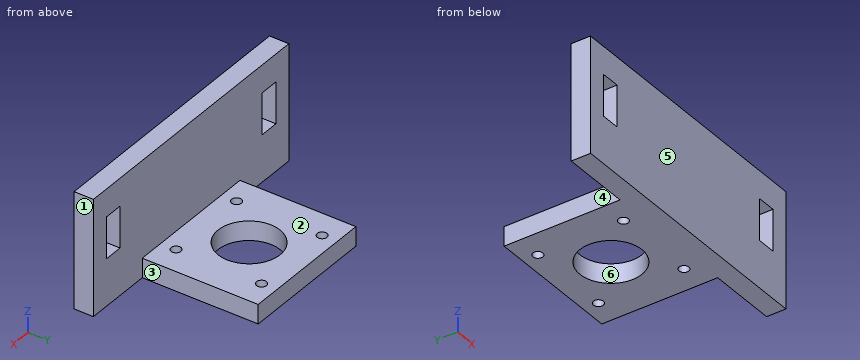
```python
from build123d import *

# Parameters (mm, degrees)
SKETCH1_W           = 50
SKETCH1_H           = 42
BOSS_EXTRUDE1_DEPTH = 49
SKETCH2_W           = 50
SKETCH2_H           = 35
CUT_EXTRUDE1_DEPTH  = 42
SKETCH3_W           = 42
SKETCH3_H           = 7
BOSS_EXTRUDE2_DEPTH = 25
SKETCH4_W           = 42
SKETCH4_H           = 7
BOSS_EXTRUDE3_DEPTH = 25
SKETCH5_R           = 11.25
SKETCH5_R_2         = 1.8
CUT_EXTRUDE2_DEPTH  = 79.268767717
SKETCH6_W           = 7
SKETCH6_H           = 15
CUT_EXTRUDE3_DEPTH  = 69.593002559


with BuildPart() as part:
    # Sketch1 → Boss-Extrude1 (new body)
    with BuildSketch(Plane(origin=(0, 0, 0), x_dir=(1, 0, 0), z_dir=(0, 1, 0))):
        Rectangle(SKETCH1_W, SKETCH1_H)
    extrude(amount=BOSS_EXTRUDE1_DEPTH)

    # Sketch2 → Cut-Extrude1 (cut)
    with BuildSketch(Plane(origin=(0, 49, 0), x_dir=(1, 0, 0), z_dir=(0, 1, 0))):
        with Locations((0, -3.5)):
            Rectangle(SKETCH2_W, SKETCH2_H)
    extrude(amount=-CUT_EXTRUDE1_DEPTH, mode=Mode.SUBTRACT)

    # Sketch3 → Boss-Extrude2 (add)
    with BuildSketch(Plane(origin=(25, 0, 0), x_dir=(0, 0, -1), z_dir=(1, 0, 0))):
        with Locations((0, 3.5)):
            Rectangle(SKETCH3_W, SKETCH3_H)
    extrude(amount=BOSS_EXTRUDE2_DEPTH)

    # Sketch4 → Boss-Extrude3 (add)
    with BuildSketch(Plane.ZY.offset(25)):
        with Locations((0, 3.5)):
            Rectangle(SKETCH4_W, SKETCH4_H)
    extrude(amount=BOSS_EXTRUDE3_DEPTH)

    # Sketch5 → Cut-Extrude2 (cut, through all)
    with BuildSketch(Plane.XY.offset(-14)):
        with Locations((0, 28)):
            Circle(SKETCH5_R)
        with Locations((-15.5, 43.5)):
            Circle(SKETCH5_R_2)
        with Locations((15.5, 43.5)):
            Circle(SKETCH5_R_2)
        with Locations((-15.5, 12.5)):
            Circle(SKETCH5_R_2)
        with Locations((15.5, 12.5)):
            Circle(SKETCH5_R_2)
    extrude(amount=-CUT_EXTRUDE2_DEPTH, mode=Mode.SUBTRACT)

    # Sketch6 → Cut-Extrude3 (cut, through all)
    with BuildSketch(Plane(origin=(0, 7, 0), x_dir=(1, 0, 0), z_dir=(0, 1, 0))):
        with Locations((-39.9, -3.5)):
            Rectangle(SKETCH6_W, SKETCH6_H)
        with Locations((39.9, -3.5)):
            Rectangle(SKETCH6_W, SKETCH6_H)
    extrude(amount=-CUT_EXTRUDE3_DEPTH, mode=Mode.SUBTRACT)


solid = part.part
```
Geometry check sheet. Reference: the model listing, model coordinates, mm. Face numbers are marked on the shaded views. A direction names the side the tool comes from. Round coordinates to 2 decimals unless told otherwise and drop trailing zeros. Order: outer loops, then holes, each group sorted by start corner. A loop starts at its lowest first (then second) coordinate and runs counter-clockwise, first axis right, second up. Notation, with made-up numbers: (86.5, -5) - (108.5, -5) arc R17 cw to (108.5, 3) - close; hole circle Ø5 at (26, 80.25). An arc over 180 degrees is marked (long way). Use a Markdown table: item, result. Add a question column.
1) Section check A-A (y = 19). Record the cut outline in (x, z).
2) Section check B-B (x = 38). Record the cut outline in (y, z).
3) Section check D-D (y = 43.5). Record the cut outline in (x, z), then the cut area to 3 significant figures.
4) Thickness scan on line 1 along X through (y, z) = (3, 10); line 2 along Y through (x, z) = (15.5, -15.75); line 3 along Y through (x, z) = (0, -16.25). Record the ranges inside material, lowest first.
5) Gauge pin test, flat ends, axial feed: P1, Ø2, axis at x = -15.5, y = 43.5, coming from the -Z side; P2, Ø10, axis at x = -39, z = -1.5, coming from the +Y side; P3, Ø5.5, axis at y = 37, z = -17, coming from the +X side. Record the tip position at first contact, or that the pin passes through.
6) Section check C-C (z = -18). Record the cut outline in (x, y), then the cut area to 3 significant figures.
7) Mould release check, pull along X, two halves, no side actions. Record for the marked faces 4, 5 and 6: released by +X, released by -X, zero draft, split by the parting line, or undercut.
8) Set-up check for the marked faces 1, 2 and 3: record each of +Z, -Z, +X, -X, +Y, -Y from which the full face is reachable in a straight line by a thin tool's end or side.
Established:
| question | item | result |
|---|---|---|
| 1 | outline | (-25, -21) - (-6.75, -21) - (-6.75, -14) - (-25, -14) - close; (6.75, -21) - (25, -21) - (25, -14) - (6.75, -14) - close |
| 2 | outline | (0, -21) - (7, -21) - (7, -4) - (0, -4) - close; (0, 11) - (7, 11) - (7, 21) - (0, 21) - close |
| 3 | outline | (-25, -21) - (-17.3, -21) - (-17.3, -14) - (-25, -14) - close; (-13.7, -21) - (13.7, -21) - (13.7, -14) - (-13.7, -14) - close; (17.3, -21) - (25, -21) - (25, -14) - (17.3, -14) - close |
| 3 | area | 300 mm2 |
| 4 | line 1 | -50 to -43.4, -36.4 to 36.4, 43.4 to 50 |
| 4 | line 2 | 0 to 10.7, 14.3 to 41.7, 45.3 to 49 |
| 4 | line 3 | 0 to 16.75, 39.25 to 49 |
| 5 | P1 | through |
| 5 | P2 | y = 7 |
| 5 | P3 | x = 25 |
| 6 | outline | (-50, 0) - (50, 0) - (50, 7) - (25, 7) - (25, 49) - (-25, 49) - (-25, 7) - (-50, 7) - close; hole circle Ø3.6 at (-15.5, 12.5); hole circle Ø3.6 at (-15.5, 43.5); hole circle Ø22.5 at (0, 28); hole circle Ø3.6 at (15.5, 12.5); hole circle Ø3.6 at (15.5, 43.5) |
| 6 | area | 2,360 mm2 |
| 7 | face 4 | released by -X |
| 7 | face 5 | zero draft |
| 7 | face 6 | undercut |
| 8 | face 1 | +Z, -Z, +X, +Y, -Y |
| 8 | face 2 | +Z, +X, -X, +Y |
| 8 | face 3 | +Z, -Z, +X, +Y |
